Work out the finished part from the listing and answer in its coordinate system (mm). A direction names the side the tool comes from. Give positions to 0.01 mm unless a question says otherwise; leave off trailing zeros. Write each loop counter-clockwise with the first axis right and the second up, starting at its lowest first coordinate (ties: lowest second). Pieces come first, ordered by that corner, then holes. Notation, with made-up numbers: (-10, 76) -> (3, 76) arc R13 ccw to (3, 88) -> close; hole circle Ø8 at (-9, 37.25). An arc over 180 degrees is marked (long way). Write item = value, one per line. Start each with the question number.
from build123d import *

# Parameters (mm, degrees)
F1_W         = 98.3519479632
F1_H         = 64.8710429668
F1_W_2       = 85.651949048
F1_H_2       = 52.1710440516
F2_DEPTH     = 50.8
F3_R         = 5.08
F4_T1_DEPTH  = 58.42
F4_S5_W      = 5.08
F4_S5_H      = 5.08
F4_T6_DEPTH  = 5.08
F4_S11_W     = 5.08
F4_S11_H     = 5.08
F4_T12_DEPTH = 5.08
F4_S17_W     = 5.08
F4_S17_H     = 5.08
F4_T18_DEPTH = 5.08
F5_T1_DEPTH  = 58.42
F5_S5_W      = 5.08
F5_S5_H      = 5.08
F5_T6_DEPTH  = 5.08


# Not quite as in the source:
# - a fillet or chamfer that OpenCascade refuses, or shapes differently, is made with other operations: its cross-section is extruded or revolved along the edge and cut away or added


with BuildPart() as f2:
    # F1 (on face) → F2 (new body)
    with BuildSketch(Plane.XZ):
        with Locations((0.1114979386, 7.887352258)):
            Rectangle(F1_W, F1_H)
        with Locations((0.1114979386, 7.887352258)):
            Rectangle(F1_W_2, F1_H_2, mode=Mode.SUBTRACT)
    extrude(amount=F2_DEPTH)

    # F3
    f3_edges = [f2.edges().sort_by_distance(p)[0] for p in [
        (0.111498, -50.8, 40.322874),
        (49.287472, -50.8, 7.887352),
        (0.111498, -50.8, -24.548169),
        (-49.064476, -50.8, 7.887352),
    ]]
    fillet(f3_edges, radius=F3_R)

    # F4: fillet of radius 5.08 on 3 edges, made by hand

    # F4_s2 → F4_t1 (cut)
    with BuildSketch(Plane.XZ.offset(-12.7)):
        with BuildLine():
            ThreePointArc((44.2074719203, 40.3228737414), (47.7995743687, 38.8349761898), (49.2874719203, 35.2428737414))
            Line((49.2874719203, 35.2428737414), (49.2874719203, 40.3228737414))
            Line((49.2874719203, 40.3228737414), (44.2074719203, 40.3228737414))
        make_face()
        with BuildLine():
            ThreePointArc((49.2874719203, -19.4681692255), (47.7995743687, -23.0602716739), (44.2074719203, -24.5481692255))
            Line((44.2074719203, -24.5481692255), (49.2874719203, -24.5481692255))
            Line((49.2874719203, -24.5481692255), (49.2874719203, -19.4681692255))
        make_face()
        with BuildLine():
            ThreePointArc((-49.064476043, -19.4681692255), (-47.5765784914, -23.0602716739), (-43.984476043, -24.5481692255))
            Line((-43.984476043, -24.5481692255), (-49.064476043, -24.5481692255))
            Line((-49.064476043, -24.5481692255), (-49.064476043, -19.4681692255))
        make_face()
    extrude(amount=F4_T1_DEPTH, mode=Mode.SUBTRACT)


with BuildPart() as f4_tool4:
    # F4_s5 → F4_t6 (new body)
    with BuildSketch(Plane.YZ.offset(-43.984476043)):
        with Locations((-48.26, -22.0081692255)):
            Rectangle(F4_S5_W, F4_S5_H)
    extrude(amount=-F4_T6_DEPTH)

    # F4_s7 → F4_t8 (revolve, cut)
    with BuildSketch(Plane(origin=(-43.984476043, -45.72, -19.4681692255), x_dir=(0, 0.7071067812, 0.7071067812), z_dir=(0, -0.7071067812, 0.7071067812))):
        with BuildLine():
            ThreePointArc((0, -5.08), (5.08, 0), (0, 5.08))
            Line((0, 5.08), (0, -5.08))
        make_face()
    revolve(axis=Axis((-43.984476043, -45.72, -19.4681692255), (-1, 0, 0)), mode=Mode.SUBTRACT)


with BuildPart() as f2_1:
    add(f2.part)

    # F4_t3: cut F4_tool4
    add(f4_tool4.part, mode=Mode.SUBTRACT)


with BuildPart() as f4_tool10:
    # F4_s11 → F4_t12 (new body)
    with BuildSketch(Plane.YZ.offset(44.2074719203)):
        with Locations((-48.26, -22.0081692255)):
            Rectangle(F4_S11_W, F4_S11_H)
    extrude(amount=F4_T12_DEPTH)

    # F4_s13 → F4_t14 (revolve, cut)
    with BuildSketch(Plane(origin=(44.2074719203, -45.72, -19.4681692255), x_dir=(0, 0.7071067812, 0.7071067812), z_dir=(0, 0.7071067812, -0.7071067812))):
        with BuildLine():
            ThreePointArc((0, -5.08), (5.08, 0), (0, 5.08))
            Line((0, 5.08), (0, -5.08))
        make_face()
    revolve(axis=Axis((44.2074719203, -45.72, -19.4681692255), (1, 0, 0)), mode=Mode.SUBTRACT)


with BuildPart() as f2_2:
    add(f2_1.part)

    # F4_t9: cut F4_tool10
    add(f4_tool10.part, mode=Mode.SUBTRACT)


with BuildPart() as f4_tool16:
    # F4_s17 → F4_t18 (new body)
    with BuildSketch(Plane.XY.offset(35.2428737414)):
        with Locations((46.7474719203, -48.26)):
            Rectangle(F4_S17_W, F4_S17_H)
    extrude(amount=F4_T18_DEPTH)

    # F4_s19 → F4_t20 (revolve, cut)
    with BuildSketch(Plane(origin=(44.2074719203, -45.72, 35.2428737414), x_dir=(-0.7071067812, 0.7071067812, 0), z_dir=(0.7071067812, 0.7071067812, 0))):
        with BuildLine():
            ThreePointArc((0, -5.08), (5.08, 0), (0, 5.08))
            Line((0, 5.08), (0, -5.08))
        make_face()
    revolve(axis=Axis((44.2074719203, -45.72, 35.2428737414), (0, 0, 1)), mode=Mode.SUBTRACT)


with BuildPart() as f2_3:
    add(f2_2.part)

    # F4_t15: cut F4_tool16
    add(f4_tool16.part, mode=Mode.SUBTRACT)

    # F5: fillet of radius 5.08 on 1 edges, made by hand

    # F5_s2 → F5_t1 (cut)
    with BuildSketch(Plane.XZ.offset(-12.7)):
        with BuildLine():
            ThreePointArc((-43.984476043, 40.3228737414), (-47.5765784914, 38.8349761898), (-49.064476043, 35.2428737414))
            Line((-49.064476043, 35.2428737414), (-49.064476043, 40.3228737414))
            Line((-49.064476043, 40.3228737414), (-43.984476043, 40.3228737414))
        make_face()
    extrude(amount=F5_T1_DEPTH, mode=Mode.SUBTRACT)


with BuildPart() as f5_tool4:
    # F5_s5 → F5_t6 (new body)
    with BuildSketch(Plane.XY.offset(35.2428737414)):
        with Locations((-46.524476043, -48.26)):
            Rectangle(F5_S5_W, F5_S5_H)
    extrude(amount=F5_T6_DEPTH)

    # F5_s7 → F5_t8 (revolve, cut)
    with BuildSketch(Plane(origin=(-43.984476043, -45.72, 35.2428737414), x_dir=(0.7071067812, 0.7071067812, 0), z_dir=(0.7071067812, -0.7071067812, 0))):
        with BuildLine():
            ThreePointArc((0, -5.08), (5.08, 0), (0, 5.08))
            Line((0, 5.08), (0, -5.08))
        make_face()
    revolve(axis=Axis((-43.984476043, -45.72, 35.2428737414), (0, 0, 1)), mode=Mode.SUBTRACT)


with BuildPart() as f2_4:
    add(f2_3.part)

    # F5_t3: cut F5_tool4
    add(f5_tool4.part, mode=Mode.SUBTRACT)


solid = f2_4.part
(1) For faces 4 (the cylindrical face through (0.729, -49.272, 38.874)), 5 (the flat face through (-42.714, -25, 8)), determine the directions among +Z, -Z, +X, -X, +Y, -Y from which every point of the face is accessible in a straight line to the end or side of a thin tool.
(2) Find the intervals of material crossed by line 1 along Z through (x, y) = (-41, -36); line 2 along X through (y, z) = (-9.5, -3); line 3 along Y through (x, z) = (25, -22), in increasing order.
(3) A cutting plane is placed at C-C, the plane y = -30. Write down the section's boundary in (x, z).
(4) A cutting plane is placed at A-A, the plane z = 29.5. Write down the section's boundary in (x, y).
(5) A cutting plane is placed at B-B, the plane x = 33. Write down the section's boundary in (y, z), then the cut area to 3 significant figures.
(6) Determine the mould class of faces 1 (the cylindrical face through (47.84, -49.27, 8.27)), 2 (the flat face through (42.937, -25, 8)), 3 (the cylindrical face through (-47.616, -22.54, -23.021)) for opening direction Z: pulls with the +Z half, pulls with the -Z half, needs draft (parallel to the pull), parting line crosses it, or undercut.
Results list:
q1.face_4 = +Z, +X, -X, -Y
q1.face_5 = +Y, -Y
q2.line_1 = -24.55 to -18.2, 33.97 to 40.32
q2.line_2 = -49.06 to -42.71, 42.94 to 49.29
q2.line_3 = -50.12 to 0
q3.outline = (-49.06, -19.47) arc R5.08 ccw to (-43.98, -24.55) -> (44.21, -24.55) arc R5.08 ccw to (49.29, -19.47) -> (49.29, 35.24) arc R5.08 ccw to (44.21, 40.32) -> (-43.98, 40.32) arc R5.08 ccw to (-49.06, 35.24) -> close; hole (-42.71, -18.2) -> (42.94, -18.2) -> (42.94, 33.97) -> (-42.71, 33.97) -> close
q4.outline = (-49.06, -45.72) arc R5.08 ccw to (-43.98, -50.8) -> (-42.71, -50.8) -> (-42.71, 0) -> (-49.06, 0) -> close; (42.94, -50.8) -> (44.21, -50.8) arc R5.08 ccw to (49.29, -45.72) -> (49.29, 0) -> (42.94, 0) -> close
q5.outline = (-50.8, -19.47) arc R5.08 ccw to (-45.72, -24.55) -> (0, -24.55) -> (0, -18.2) -> (-50.8, -18.2) -> close; (-50.8, 33.97) -> (0, 33.97) -> (0, 40.32) -> (-45.72, 40.32) arc R5.08 ccw to (-50.8, 35.24) -> close
q5.area = 634 mm²
q6.face_1 = needs draft
q6.face_2 = undercut
q6.face_3 = pulls with the -Z half
